Could you check a few things on this model? Use its own coordinates, in mm. A direction names the side the tool comes from. Give positions to 0.01 mm unless a question says otherwise; leave off trailing zeros. Loops run counter-clockwise (first coordinate to the right, second up) from the corner with the lowest first, then second, coordinate; pieces in that order, holes last. Notation, with made-up numbers: (52, 60.25) -> (72, 60.25) arc R14 cw to (72, 82.25) -> close; hole circle Ø10 at (6, -9.75). An arc over 180 degrees is marked (long way). Put each result on its own line as item: value.
```python
from build123d import *

# Parameters (mm, degrees)
F1_DEPTH = 15
F2_R     = 1
F3_DEPTH = 17
F5_W     = 2
F5_H     = 18.8568213596
F6_DEPTH = 12.5


with BuildPart() as f1:
    # F0 (on Right) → F1 (new body, symmetric)
    with BuildSketch(Plane.YZ):
        with BuildLine():
            Line((2.5, 0), (1, 0))
            ThreePointArc((1, 0), (0.7071067812, -0.7071067812), (0, -1))
            Line((0, -1), (0, -2.5))
            ThreePointArc((0, -2.5), (1.767766953, -1.767766953), (2.5, 0))
        make_face()
        with BuildLine():
            ThreePointArc((0, -1), (-0.7071067812, 0.7071067812), (1, 0))
            Line((1, 0), (2.5, 0))
            ThreePointArc((2.5, 0), (2.4637418621, 0.4242358271), (2.3560191704, 0.8361660533))
            ThreePointArc((2.3560191704, 0.8361660533), (2.32783074, 0.9037284298), (2.3030468589, 0.9726125467))
            ThreePointArc((2.3030468589, 0.9726125467), (-2.0834504274, 1.3817504538), (0, -2.5))
            Line((0, -2.5), (0, -1))
        make_face()
        with BuildLine():
            Line((3.3880661343, 0), (2.5, 0))
            ThreePointArc((2.5, 0), (1.767766953, -1.767766953), (0, -2.5))
            Line((0, -2.5), (19.75, -2.5))
            ThreePointArc((19.75, -2.5), (18.5, -1.25), (19.75, 0))
            Line((19.75, 0), (3.3880661343, 0))
        make_face()
        with BuildLine():
            ThreePointArc((2.3560191704, 0.8361660533), (2.4637418621, 0.4242358271), (2.5, 0))
            Line((2.5, 0), (3.3880661343, 0))
            ThreePointArc((3.3880661343, 0), (2.7720196419, 0.2946285479), (2.3560191704, 0.8361660533))
        make_face()
        with BuildLine():
            ThreePointArc((2.3030468589, 0.9726125467), (2.32783074, 0.9037284298), (2.3560191704, 0.8361660533))
            ThreePointArc((2.3560191704, 0.8361660533), (2.3305318015, 0.9047770567), (2.3030468589, 0.9726125467))
        make_face()
        with BuildLine():
            ThreePointArc((19.75, 0), (18.5, -1.25), (19.75, -2.5))
            Line((19.75, -2.5), (19.75, 0))
        make_face()
        with BuildLine():
            Line((19.75, 0), (19.75, -2.5))
            ThreePointArc((19.75, -2.5), (20.6338834765, -2.1338834765), (21, -1.25))
            ThreePointArc((21, -1.25), (20.6338834765, -0.3661165235), (19.75, 0))
        make_face()
    extrude(amount=F1_DEPTH, both=True)

    # F2 (on Right) → F3 (join, symmetric)
    with BuildSketch(Plane.YZ):
        Circle(F2_R)
    extrude(amount=F3_DEPTH, both=True)

    # F4 (on Top) + F5 (on Top) → F6 (cut, symmetric)
    with BuildSketch(Plane.XY):
        Polygon((-14.564535037, -3.0443312038), (-17, 0), (-18.738245276, 0), (-18.738245276, -3.0443312038), align=None)
        Polygon((18.738245276, -3.0443312038), (18.738245276, 0), (17, 0), (14.564535037, -3.0443312038), align=None)
    with BuildSketch(Plane.XY):
        with Locations((-10, 3.5715893202)):
            Rectangle(F5_W, F5_H)
        with Locations((10, 3.5715893202)):
            Rectangle(F5_W, F5_H)
    extrude(amount=F6_DEPTH, both=True, mode=Mode.SUBTRACT)


solid = f1.part
```
1. Thinking about a two-plate mould opening in X: for faces 1 (the face through (-16, 1, 0)), 2 (the face through (16.694, -0.382, -0.014)), 3 (the face through (-10, 13, -1)), which applies, pulls with the +X half, pulls with the -X half, needs draft (parallel to the pull), parting line crosses it, or undercut?
Recorded:
face 1: needs draft
face 2: pulls with the +X half
face 3: undercut
2. If we section it at B-B (x = -14): List the corners of the cut face in (y, z) for me, then the cut area to 3 significant figures.
Recorded:
outline: (0, -2.5) -> (19.75, -2.5) arc R1.25 ccw to (19.75, 0) -> (3.39, 0) arc R1.47 cw to (2.36, 0.84) arc R2.5 ccw (long way) to start
area: 66.8 mm^2
3. I'm going to push flat-ended pins straight in: pin 1 (1.5 mm diameter, centred on y = 4, z = 1, fed in from +X); pin 2 (1.6 mm diameter, centred on x = -9.5, z = -1, fed in from -Y); pin 3 (2.5 mm diameter, centred on y = 15, z = 0.5, fed in from +X); pin 4 (1.5 mm diameter, centred on x = -9, z = 0, fed in from +Y). Where does each tip first touch, or does it pass through?
Recorded:
pin 1: passes through
pin 2: stops at y = -2.47
pin 3: stops at x = 15
pin 4: stops at y = 20.9
4. For faces 4 (the face through (-16.68, -0.4, -0.01)), 5 (the face through (11, 3, -1)), 6 (the face through (0, 10, -2.5)), 7 (the face through (0, 12, 0)), 8 (the face through (16, 1, 0)), which set-ups out of +Z, -Z, +X, -X, +Y, -Y let a thin tool reach every point of the face, with its end or its side?
Recorded:
face 4: +Z, -Z, -X, -Y
face 5: +Z, -Z, -Y
face 6: -Z, +X, -X, +Y, -Y
face 7: +Z, +X, -X, +Y
face 8: +X
5. I need wall thicknesses on line 1 (X direction, y = 0.25, z = -2.3); line 2 (Z direction, x = -8, y = 15.5); line 3 (X direction, y = 18, z = -1.7). Which ranges of each line are inside material? Lowest first, please.
Recorded:
line 1: x = -15 to -11, -9 to 9, 11 to 15
line 2: z = -2.5 to 0
line 3: x = -15 to 15
6. If we section it at A-A (y = 5.75): List the corners of the cut face in (x, z) for me, then the cut area to 3 significant figures.
Recorded:
outline: (-15, -2.5) -> (-11, -2.5) -> (-11, 0) -> (-15, 0) -> close; (-9, -2.5) -> (9, -2.5) -> (9, 0) -> (-9, 0) -> close; (11, -2.5) -> (15, -2.5) -> (15, 0) -> (11, 0) -> close
area: 65.0 mm^2
